Input: part model. Units: mm. Frame: model coordinates. Round coordinates to 2 decimals unless told otherwise and drop trailing zeros. Order: outer loops, then holes, each group sorted by start corner. A loop starts at its lowest first (then second) coordinate and runs counter-clockwise, first axis right, second up. Notation, with made-up numbers: (11, 6.25) -> (62, 6.25) arc R28 cw to (62, 27.25) -> close; hole circle Ø7 at (40, -13.5). An arc over 180 degrees is marked (long way). Answer as CSV lines item,"result". Start each with the question number.
1) Section query D-D, the plane y = -18. Output: boundary loops of the cut face in (x, z), and give its area (3 significant figures).
2) Section query B-B, the plane z = 0.5. State how many separate pieces and enclosed holes the cut face has, and give its area (3 significant figures).
3) Mould query, pull axis X, two halves, no side actions, for faces 1 (the face through (29.386, -10.669, 1.521)), 2 (the face through (92.603, -34.098, 1.521)), 3 (the face through (17.742, -13.372, 1.521)), 4 (the face through (66.613, -34.109, 1.521)). Classes: +X half, -X half, draft (parallel to the pull), parting line (faces both ways), or undercut.
4) Section query A-A, the plane x = 69. Output: boundary loops of the cut face in (y, z).
5) Section query C-C, the plane y = -31.5. Output: boundary loops of the cut face in (x, z).
6) Line query: L1, parallel to X at y = -33, z = 0.95; L2, parallel to Y at x = 71.5, z = 2.15; L3, parallel to X at y = -57.5, z = 1.7. Output: solid intervals per line, ascending.
```python
from build123d import *

# Parameters (mm, degrees)
SKETCH1_W           = 95
SKETCH1_H           = 100
BOSS_EXTRUDE1_DEPTH = 3
CUT_EXTRUDE3_DEPTH  = 3
SKETCH5_R           = 2.43527257
SKETCH5_R_2         = 7
SKETCH5_R_3         = 3.5
CUT_EXTRUDE4_DEPTH  = 3


with BuildPart() as part:
    # Sketch1 → Boss-Extrude1 (new body)
    with BuildSketch(Plane.XY):
        with Locations((47.5, -50)):
            Rectangle(SKETCH1_W, SKETCH1_H)
    extrude(amount=BOSS_EXTRUDE1_DEPTH)

    # Sketch4 → Cut-Extrude3 (cut)
    with BuildSketch(Plane.XY.offset(3)):
        Polygon((33.610991992, -100), (62.120295215, -100), (95, -100), (95, 0), (0, 0), (0, -100), align=None)
        with BuildLine():
            Line((78.778954762, -5.219976488), (84.72769663, -19.012180272))
            ThreePointArc((84.72769663, -19.012180272), (92.605897001, -34.348605074), (84.838305738, -49.741346636))
            Line((84.838305738, -49.741346636), (64.0242126, -95.787997202))
            Line((64.0242126, -95.787997202), (31.934866328, -95.787997202))
            Line((31.934866328, -95.787997202), (14.049192276, -50.842376041))
            ThreePointArc((14.049192276, -50.842376041), (6.549499619, -35.317345386), (14.692273517, -20.119740309))
            Line((14.692273517, -20.119740309), (20.879119665, -6.432689868))
            ThreePointArc((20.879119665, -6.432689868), (22.012480764, -5.130871888), (23.675593701, -4.669035561))
            Line((23.675593701, -4.669035561), (75.890580945, -3.41108885))
            ThreePointArc((75.890580945, -3.41108885), (75.952006311, -3.408979239), (76.013462004, -3.408128439))
            ThreePointArc((76.013462004, -3.408128439), (77.66832232, -3.898714586), (78.778954762, -5.219976488))
        make_face(mode=Mode.SUBTRACT)
    extrude(amount=-CUT_EXTRUDE3_DEPTH, mode=Mode.SUBTRACT)

    # Sketch5 → Cut-Extrude4 (cut)
    with BuildSketch(Plane.XY.offset(3)):
        with Locations((54.906624154, -84.449867327)):
            Circle(SKETCH5_R)
        with Locations((47.979539464, -91.376952018)):
            Circle(SKETCH5_R)
        with Locations((41.052454773, -84.449867327)):
            Circle(SKETCH5_R)
        with Locations((47.979539464, -77.522782636)):
            Circle(SKETCH5_R)
        with Locations((73.606020085, -34.416994806)):
            Circle(SKETCH5_R_2)
        with Locations((25.545338638, -35.714963215)):
            Circle(SKETCH5_R_2)
        with Locations((25.043084538, -59.70970724)):
            Circle(SKETCH5_R_3)
        with Locations((26.047592738, -11.72021919)):
            Circle(SKETCH5_R_3)
        with Locations((73.692407115, -58.416839333)):
            Circle(SKETCH5_R_3)
        with Locations((73.519633055, -10.41715028)):
            Circle(SKETCH5_R_3)
    extrude(amount=-CUT_EXTRUDE4_DEPTH, mode=Mode.SUBTRACT)


solid = part.part
```
Findings:
1,outline,"(15.65, 0) -> (84.29, 0) -> (84.29, 3) -> (15.65, 3) -> close"
1,area,"206 mm^2"
2,separate pieces,"1"
2,enclosed holes,"10"
2,area,"5,280 mm^2"
3,face 1,"undercut"
3,face 2,"+X half"
3,face 3,"-X half"
3,face 4,"undercut"
4,outline,"(-84.78, 0) -> (-39.69, 0) -> (-39.69, 3) -> (-84.78, 3) -> close; (-29.15, 0) -> (-3.58, 0) -> (-3.58, 3) -> (-29.15, 3) -> close"
5,outline,"(7.02, 0) -> (19.96, 0) -> (19.96, 3) -> (7.02, 3) -> close; (31.13, 0) -> (67.24, 0) -> (67.24, 3) -> (31.13, 3) -> close; (79.97, 0) -> (92.38, 0) -> (92.38, 3) -> (79.97, 3) -> close"
6,L1,"x = 6.74 to 19.09, 32 to 66.75, 80.46 to 92.55"
6,L2,"y = -79.25 to -61.15, -55.69 to -41.09, -27.74 to -13.28, -7.56 to -3.52"
6,L3,"x = 16.7 to 22.33, 27.76 to 70.31, 77.07 to 81.33"
